Autodesk Inventor part; units mm, degrees
ref_plane "YZ Plane" through (0, 0, 0) normal (1, 0, 0) x (0, 1, 0)
ref_plane "XZ Plane" through (0, 0, 0) normal (0, 1, 0) x (-1, 0, 0)
ref_plane "XY Plane" through (0, 0, 0) normal (0, 0, 1) x (1, 0, 0)
sketch "Sketch1" plane through (0, 0, 0) normal (0, 0, 1) x (1, 0, 0)
  line L0 (0, 0) -> (160, 0)
  line L1 (160, 0) -> (160, 160)
  line L2 (160, 160) -> (0, 160)
  line L3 (0, 160) -> (0, 0)
  dimension "d0" = 160
  dimension "d1" = 160
extrude "Extrusion1" add sketch "Sketch1" along normal blind 10
sketch "Sketch2" plane through (0, 0, 10) normal (0, 0, 1) x (1, 0, 0)
  line L0 (0, 0) -> (160, 0)
  line L1 (0, 0) -> (15, 0)
  line L2 (15, 0) -> (15, 15)
  line L3 (160, 160) -> (0, 160)
  line L4 (0, 160) -> (15, 160)
  line L5 (15, 160) -> (15, 145)
  line L6 (160, 0) -> (160, 160)
  line L7 (160, 160) -> (145, 160)
  line L8 (145, 160) -> (145, 143.5)
  line L9 (160, 0) -> (160, 15)
  line L10 (160, 15) -> (145, 15)
  circle A0 centre (15, 145) radius 7.5
  circle A1 centre (145, 143.5) radius 7.5
  circle A2 centre (145, 15) radius 7.5
  circle A3 centre (15, 15) radius 7.5
  dimension "d4" = 15
  dimension "d5" = 15
  dimension "d6" = 15
  dimension "d7" = 15
  dimension "d8" = 15
  dimension "d9" = 16.5
  dimension "d10" = 15
  dimension "d11" = 15
  dimension "d12" = 15
  dimension "d13" = 15
  dimension "d14" = 15
  dimension "d15" = 15
extrude "Extrusion2" cut sketch "Sketch2" against normal blind 10
sketch "Sketch3" plane through (0, 0, 10) normal (0, 0, 1) x (1, 0, 0)
  line L0 (0, 160) -> (0, 0)
  line L1 (0, 0) -> (80, 0)
  line L2 (0, 0) -> (160, 0)
  line L3 (80, 0) -> (0, 0)
  line L4 (0, 0) -> (80, 0)
  dimension "d18" = 80
  dimension "d19" = 80
  dimension "d20" = 80
sketch "Sketch4" plane through (0, 0, 10) normal (0, 0, 1) x (1, 0, 0)
  line L0 (0, 0) -> (0, 80)
  line L1 (0, 160) -> (0, 0)
  line L2 (0, 80) -> (80, 80)
  circle A0 centre (80, 80) radius 7.5
  dimension "d21" = 80
  dimension "d22" = 80
  dimension "d23" = 15
extrude "Extrusion3" cut sketch "Sketch4" against normal blind 10
sketch "Sketch5" plane through (0, 0, 10) normal (0, 0, 1) x (1, 0, 0)
  line L0 (160, 0) -> (160, 160)
  line L1 (160, 0) -> (160, 80)
  line L2 (160, 80) -> (125, 80)
  circle A0 centre (125, 80) radius 30
  point P0 (0, 0)
  dimension "d26" = 80
  dimension "d27" = 35
  dimension "d28" = 60
extrude "Extrusion4" cut sketch "Sketch5" against normal blind 10
properties part number "100"
The model under review builds one solid part; all positions refer to its coordinate system, in mm. Coordinates: 2 decimals unless noted, no trailing zeros. Write each loop counter-clockwise with the first axis right and the second up, starting at its lowest first coordinate (ties: lowest second). Pieces come first, ordered by that corner, then holes. Notation, with made-up numbers: (39.25, 63) -> (54.25, 63) arc R17 cw to (54.25, 78) -> close; hole circle Ø4 at (14.25, 74). An arc over 180 degrees is marked (long way). One line per item, written item: value. Start each with the question number.
Q1. Add section A-A, the plane y = 15. Give the boundary of the cut face in (x, z).
Q2. To check wall thickness, follow probe 1 along X at (y, z) = (80.5, 4.5); probe 2 along Y at (x, z) = (125, 6); probe 3 along X at (y, z) = (145.5, 2.5). State the ranges of each line that lie inside material, in increasing order.
Q3. Add section D-D, the plane x = 80. Give the boundary of the cut face in (y, z), then the cut area to 3 significant figures.
Q4. The part is to be moulded in two halves that separate along X. For faces 1 (the face through (160, 79, 5)), 2 (the face through (61, 81, 10)), 3 (the face through (152.154, 17.253, 5.07)), say which applies: +X half, -X half, draft (parallel to the pull), parting line (faces both ways), or undercut.
Q5. Add section C-C, the plane z = 1.5. Give the boundary of the cut face in (x, y).
Q6. Clearance check with a flat-ended pin moving along its axis: P1, Ø24, axis at x = 145, y = 15, coming from the +Z side. State where the tip first meets the part, or that it passes through.
Response:
1. outline: (0, 0) -> (7.5, 0) -> (7.5, 10) -> (0, 10) -> close; (22.5, 0) -> (137.5, 0) -> (137.5, 10) -> (22.5, 10) -> close; (152.5, 0) -> (160, 0) -> (160, 10) -> (152.5, 10) -> close
2. probe 1: 0 to 72.52, 87.48 to 95, 155 to 160
2. probe 2: 0 to 50, 110 to 160
2. probe 3: 0 to 7.52, 22.48 to 137.77, 152.23 to 160
3. outline: (0, 0) -> (72.5, 0) -> (72.5, 10) -> (0, 10) -> close; (87.5, 0) -> (160, 0) -> (160, 10) -> (87.5, 10) -> close
3. area: 1,450 mm²
4. face 1: +X half
4. face 2: draft
4. face 3: undercut
5. outline: (0, 0) -> (160, 0) -> (160, 160) -> (0, 160) -> close; hole circle Ø15 at (15, 15); hole circle Ø15 at (15, 145); hole circle Ø15 at (80, 80); hole circle Ø60 at (125, 80); hole circle Ø15 at (145, 15); hole circle Ø15 at (145, 143.5)
6. P1: z = 10
